Autodesk Inventor part; units mm, degrees
ref_plane "YZ Plane" through (0, 0, 0) normal (1, 0, 0) x (0, 1, 0)
ref_plane "XZ Plane" through (0, 0, 0) normal (0, 1, 0) x (-1, 0, 0)
ref_plane "XY Plane" through (0, 0, 0) normal (0, 0, 1) x (1, 0, 0)
sketch "Sketch1" plane through (0, 0, 0) normal (0, 1, 0) x (-1, 0, 0)
  line L0 (0, 0) -> (177.8, 0)
  line L1 (177.8, 0) -> (177.8, 88.9)
  line L2 (177.8, 88.9) -> (0, 88.9)
  line L3 (0, 88.9) -> (0, 0)
  line L4 (9.3218, 3.175) -> (16.0782, 3.175)
  line L5 (16.0782, 3.175) -> (16.0782, 85.725)
  line L6 (16.0782, 85.725) -> (9.3218, 85.725)
  line L7 (9.3218, 85.725) -> (9.3218, 3.175)
  line L8 (9.3218, 3.175) -> (16.0782, 85.725) construction
  line L9 (16.0782, 3.175) -> (9.3218, 85.725) construction
  line L10 (168.4782, 3.175) -> (161.7218, 3.175)
  line L11 (161.7218, 3.175) -> (161.7218, 85.725)
  line L12 (161.7218, 85.725) -> (168.4782, 85.725)
  line L13 (168.4782, 85.725) -> (168.4782, 3.175)
  line L14 (168.4782, 3.175) -> (161.7218, 85.725) construction
  line L15 (161.7218, 3.175) -> (168.4782, 85.725) construction
  point P0 (12.7, 44.45)
  point P1 (165.1, 44.45)
  dimension "d0" = 177.8
  dimension "d1" = 88.9
  dimension "d2" = 6.7564
  dimension "d3" = 82.55
  dimension "d4" = 6.7564
  dimension "d5" = 82.55
extrude "Extrusion1" add sketch "Sketch1" along normal blind 6.35
sketch "Sketch2" plane through (0, 6.35, 0) normal (0, 1, 0) x (1, 0, 0)
  line L0 (-155.575, 0) -> (-22.225, 0)
  line L1 (-22.225, 0) -> (-22.225, -88.9)
  line L2 (-22.225, -88.9) -> (-155.575, -88.9)
  line L3 (-155.575, -88.9) -> (-155.575, 0)
  line L4 (-155.575, 0) -> (-22.225, -88.9) construction
  line L5 (-22.225, 0) -> (-155.575, -88.9) construction
  point P0 (-88.9, -44.45)
  dimension "d8" = 133.35
  dimension "d9" = 88.9
extrude "Extrusion2" add sketch "Sketch2" along normal blind 50.8
sketch "Sketch3" plane through (0, 57.15, 0) normal (0, 1, 0) x (1, 0, 0)
  line L0 (-149.9, -64.45) -> (-27.9, -64.45)
  line L1 (-27.9, -64.45) -> (-27.9, -24.45)
  line L2 (-27.9, -24.45) -> (-149.9, -24.45)
  line L3 (-149.9, -24.45) -> (-149.9, -64.45)
  line L4 (-149.9, -64.45) -> (-27.9, -24.45) construction
  line L5 (-27.9, -64.45) -> (-149.9, -24.45) construction
  point P0 (0, 0)
  point P1 (-88.9, -44.45)
  dimension "d12" = 122
  dimension "d13" = 40
hole "Hole1" at (-149.9, 57.15, 24.45) at (-149.9, 57.15, 64.45) at (-27.9, 57.15, 24.45) at (-27.9, 57.15, 64.45) direction (0, -1, 0) diameter 2.4638 depth 12.7 tip angle 118
properties part number "MPB561LaserMount"
CAD build for the part. Positions are in the model's coordinates, mm. A direction names the side the tool comes from. Coordinates: 2 decimals unless noted, no trailing zeros. Write each loop counter-clockwise with the first axis right and the second up, starting at its lowest first coordinate (ties: lowest second). Pieces come first, ordered by that corner, then holes.
(1) Flat gauge pins, fed straight in: pin 1 (11 mm diameter, centred on x = -14, z = 60.5, fed in from +Y); pin 2 (4 mm diameter, centred on y = 43, z = 13, fed in from -X) (3 decimals). Where does each tip first touch, or does it go through?
(2) 3-axis set-ups, long thin cutter, end or side, ignore diameter. For faces 4 (the face through (-90, 28, 88.9)), 5 (the face through (0, 3, 45)), 6 (the face through (-169, 6.35, 45)), 7 (the face through (-165, 3, 3.175)), 8 (the face through (-22.225, 31, 44)): which of +Z, -Z, +X, -X, +Y, -Y reach the whole face in a straight line?
(3) Cut at A-A, the plane z = 30. List the corners of the cut face in (x, y) (3 decimals).
(4) Two-plate mould, pull along Z, no slides. Class faces 1 (the face through (-90, 57.15, 44)), 2 (the face through (-88, 28, 0)), 3 (the face through (-13, 3, 3.175)): +Z half, -Z half, draft (parallel to the pull), parting line (faces both ways), or undercut.
(5) Cut at B-B, the plane y = 54.5. List the corners of the cut face in (x, z) (3 decimals), and give its area (3 significant figures).
(6) Drill centre lines: probe 1 along Z at (x, y) = (-149.9, 53.5); probe 2 along X at (y, z) = (54, 24.45) (3 decimals); probe 3 along X at (y, z) = (54, 24) (3 decimals). Where is each one in solid material? Low to high.
(7) Cut at C-C, the plane y = 9. List the corners of the cut face in (x, z) (3 decimals).
Geometry says:
1. pin 1: stops at y = 6.35
1. pin 2: stops at x = -155.575
2. face 4: +Z, +X, -X, +Y, -Y
2. face 5: +Z, -Z, +X, +Y, -Y
2. face 6: +Z, -Z, -X, +Y
2. face 7: +Y, -Y
2. face 8: +Z, -Z, +X, +Y
3. outline: (-177.8, 0) - (-168.478, 0) - (-168.478, 6.35) - (-177.8, 6.35) - close; (-161.722, 0) - (-16.078, 0) - (-16.078, 6.35) - (-22.225, 6.35) - (-22.225, 57.15) - (-155.575, 57.15) - (-155.575, 6.35) - (-161.722, 6.35) - close; (-9.322, 0) - (0, 0) - (0, 6.35) - (-9.322, 6.35) - close
4. face 1: draft
4. face 2: -Z half
4. face 3: undercut
5. outline: (-155.575, 0) - (-22.225, 0) - (-22.225, 88.9) - (-155.575, 88.9) - close; hole circle Ø2.464 at (-149.9, 24.45); hole circle Ø2.464 at (-149.9, 64.45); hole circle Ø2.464 at (-27.9, 24.45); hole circle Ø2.464 at (-27.9, 64.45)
5. area: 11,800 mm2
6. probe 1: z = 0 to 23.22, 25.68 to 63.22, 65.68 to 88.9
6. probe 2: x = -155.575 to -151.132, -148.668 to -29.132, -26.668 to -22.225
6. probe 3: x = -155.575 to -151.047, -148.753 to -29.047, -26.753 to -22.225
7. outline: (-155.575, 0) - (-22.225, 0) - (-22.225, 88.9) - (-155.575, 88.9) - close
